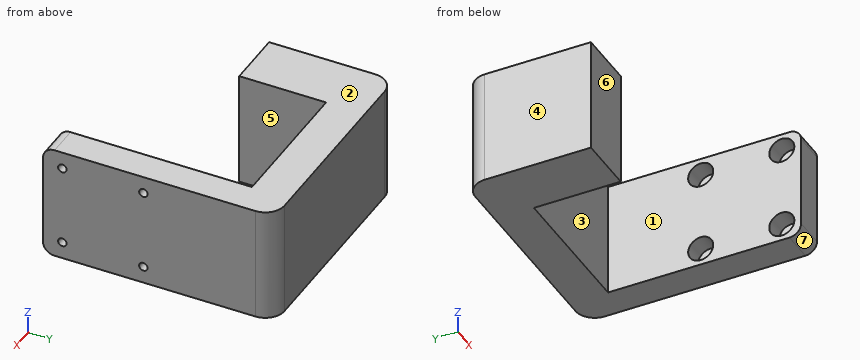
from build123d import *

# Parameters (mm, degrees)
EXTRUDE_1_DEPTH     = 30
SKETCH_2_R          = 1.1
CUT_EXTRUDE_1_DEPTH = 69.494817322
FILLET_1_R          = 3
SKETCH_3_R          = 3.25
CUT_EXTRUDE_2_DEPTH = 5


with BuildPart() as part:
    # ｽｹｯﾁ1 → ﾎﾞｽ - 押し出し1 (new body)
    with BuildSketch(Plane.XY):
        with BuildLine():
            ThreePointArc((-15, 27.5), (-13.535533906, 31.035533906), (-10, 32.5))
            Line((-10, 32.5), (40.3, 32.5))
            ThreePointArc((40.3, 32.5), (43.835533906, 31.035533906), (45.3, 27.5))
            Line((45.3, 27.5), (45.3, -27.5))
            Line((45.3, -27.5), (37.3, -27.5))
            Line((37.3, -27.5), (37.3, 22.5))
            Line((37.3, 22.5), (0, 22.5))
            Line((0, 22.5), (0, 0))
            Line((0, 0), (-15, 0))
            Line((-15, 0), (-15, 27.5))
        make_face()
    extrude(amount=EXTRUDE_1_DEPTH)

    # ｽｹｯﾁ2 → ｶｯﾄ - 押し出し1 (cut, through all)
    with BuildSketch(Plane.ZY.offset(-37.3)):
        with Locations(Location((4.5, -22.5, 0), (0, 0, 270))):
            Circle(SKETCH_2_R)
        with Locations(Location((25.5, -22.5, 0), (0, 0, 270))):
            Circle(SKETCH_2_R)
        with Locations(Location((4.5, -1.5, 0), (0, 0, 270))):
            Circle(SKETCH_2_R)
        with Locations(Location((25.5, -1.5, 0), (0, 0, 270))):
            Circle(SKETCH_2_R)
    extrude(amount=-CUT_EXTRUDE_1_DEPTH, mode=Mode.SUBTRACT)

    # ﾌｨﾚｯﾄ1
    fillet_1_edges = [part.edges().sort_by_distance(p)[0] for p in [
        (41.3, -27.5, 0),
        (41.3, -27.5, 30),
    ]]
    fillet(fillet_1_edges, radius=FILLET_1_R)

    # ｽｹｯﾁ3 → ｶｯﾄ - 押し出し2 (cut)
    with BuildSketch(Plane.ZY.offset(-37.3)):
        with Locations(Location((4.5, -22.5, 0), (0, 0, 270))):
            Circle(SKETCH_3_R)
        with Locations(Location((25.5, -22.5, 0), (0, 0, 270))):
            Circle(SKETCH_3_R)
        with Locations(Location((4.5, -1.5, 0), (0, 0, 270))):
            Circle(SKETCH_3_R)
        with Locations(Location((25.5, -1.5, 0), (0, 0, 270))):
            Circle(SKETCH_3_R)
    extrude(amount=-CUT_EXTRUDE_2_DEPTH, mode=Mode.SUBTRACT)


solid = part.part
Geometry check sheet. Reference: the model listing, model coordinates, mm. Face numbers are marked on the shaded views. A direction names the side the tool comes from. Round coordinates to 2 decimals unless told otherwise and drop trailing zeros. Loops run counter-clockwise (first coordinate to the right, second up) from the corner with the lowest first, then second, coordinate; pieces in that order, holes last.
Item 1: Gauge pin test, flat ends, axial feed: pin 1 (8 mm diameter, centred on x = 21.5, z = 7.5, fed in from -Y); pin 2 (7.5 mm diameter, centred on y = -22.5, z = 4.5, fed in from -X); pin 3 (4.5 mm diameter, centred on x = -6.5, z = 15.5, fed in from -Y). Record the tip position at first contact, or that the pin passes through.
Item 2: Cross-section at D-D on z = 11.25. Record the boundary of the cut face in (x, y), then the cut area to 3 significant figures.
Item 3: Thickness scan on line 1 (Z direction, x = 43.85, y = -1.5); line 2 (X direction, y = 15.5, z = 21.25); line 3 (Z direction, x = 44, y = -22). Record the ranges inside material, lowest first.
Item 4: Cross-section at A-A on z = 4.5. Record the boundary of the cut face in (x, y), then the cut area to 3 significant figures.
Item 5: Access from +Z, -Z, +X, -X, +Y, -Y to the whole of each face (thin tool, end or side, straight path). Record for the marked faces 5, 6 and 7.
Item 6: Cross-section at B-B on y = -22.5. Record the boundary of the cut face in (x, z).
Item 7: Cross-section at C-C on y = 13. Record the boundary of the cut face in (x, z).
Item 8: Mould release check, pull along X, two halves, no side actions. Record for the marked faces 1, 2, 3 and 4: pulls with the +X half, pulls with the -X half, needs draft (parallel to the pull), parting line crosses it, or undercut.
Answer sheet:
1. pin 1: stops at y = 22.5
1. pin 2: stops at x = 37.3
1. pin 3: stops at y = 0
2. outline: (-15, 0) - (0, 0) - (0, 22.5) - (37.3, 22.5) - (37.3, -27.5) - (45.3, -27.5) - (45.3, 27.5) arc R5 ccw to (40.3, 32.5) - (-10, 32.5) arc R5 ccw to (-15, 27.5) - close
2. area: 1,330 mm2
3. line 1: z = 0 to 3.4, 5.6 to 24.4, 26.6 to 30
3. line 2: x = -15 to 0, 37.3 to 45.3
3. line 3: z = 0 to 3.52, 5.48 to 24.52, 26.48 to 30
4. outline: (-15, 0) - (0, 0) - (0, 22.5) - (37.3, 22.5) - (37.3, 1.75) - (42.3, 1.75) - (42.3, -0.4) - (45.3, -0.4) - (45.3, 27.5) arc R5 ccw to (40.3, 32.5) - (-10, 32.5) arc R5 ccw to (-15, 27.5) - close; (37.3, -27.5) - (45.3, -27.5) - (45.3, -23.6) - (42.3, -23.6) - (42.3, -25.75) - (37.3, -25.75) - close; (37.3, -19.25) - (42.3, -19.25) - (42.3, -21.4) - (45.3, -21.4) - (45.3, -2.6) - (42.3, -2.6) - (42.3, -4.75) - (37.3, -4.75) - close
4. area: 1,250 mm2
5. face 5: +Z, -Z, -Y
5. face 6: +Z, -Z, -X, -Y
5. face 7: -Z, +X, -X, -Y
6. outline: (37.3, 0) - (45.3, 0) - (45.3, 3.4) - (42.3, 3.4) - (42.3, 1.25) - (37.3, 1.25) - close; (37.3, 7.75) - (42.3, 7.75) - (42.3, 5.6) - (45.3, 5.6) - (45.3, 24.4) - (42.3, 24.4) - (42.3, 22.25) - (37.3, 22.25) - close; (37.3, 28.75) - (42.3, 28.75) - (42.3, 26.6) - (45.3, 26.6) - (45.3, 30) - (37.3, 30) - close
7. outline: (-15, 0) - (0, 0) - (0, 30) - (-15, 30) - close; (37.3, 0) - (45.3, 0) - (45.3, 30) - (37.3, 30) - close
8. face 1: undercut
8. face 2: needs draft
8. face 3: undercut
8. face 4: pulls with the -X half
